from build123d import *

# Parameters (mm, degrees)
SKETCH2_W               = 3.8
SKETCH2_H               = 2.5
CUT_EXTRUDE1_DEPTH      = 10
CUT_EXTRUDE1_DEPTH_BACK = 7.25
SKETCH3_R               = 0.4
CUT_EXTRUDE2_DEPTH      = 7.25
CUT_EXTRUDE2_DEPTH_BACK = 7.25


with BuildPart() as part:
    # Sketch1 → Revolve1 (revolve)
    with BuildSketch(Plane.XY):
        with BuildLine():
            Line((0, 8.3), (0, 5.6))
            ThreePointArc((0, 5.6), (-2.071834936, 5.23939732), (-3.9, 4.2))
            Line((-3.9, 4.2), (-3.9, 0))
            Line((-3.9, 0), (-6.25, 0))
            Line((-6.25, 0), (-6.25, 4.6))
            Line((-6.25, 4.6), (-5.25, 4.6))
            ThreePointArc((-5.25, 4.6), (-3.211405456, 7.282061795), (0, 8.3))
        make_face()
    revolve(axis=Axis((0, 0, 0), (0, 1, 0)))

    # Sketch2 → Cut-Extrude1 (cut, two sides)
    with BuildSketch(Plane(origin=(0, 0, 0), x_dir=(0, 0, -1), z_dir=(1, 0, 0))) as cut_extrude1_sk:
        with Locations((0, 1.25)):
            Rectangle(SKETCH2_W, SKETCH2_H)
    extrude(amount=CUT_EXTRUDE1_DEPTH, mode=Mode.SUBTRACT)
    extrude(cut_extrude1_sk.sketch, amount=-CUT_EXTRUDE1_DEPTH_BACK, mode=Mode.SUBTRACT)

    # Sketch3 → Cut-Extrude2 (cut, two sides)
    with BuildSketch(Plane.XY) as cut_extrude2_sk:
        with Locations((0, 1.5)):
            Circle(SKETCH3_R)
    extrude(amount=CUT_EXTRUDE2_DEPTH, mode=Mode.SUBTRACT)
    extrude(cut_extrude2_sk.sketch, amount=-CUT_EXTRUDE2_DEPTH_BACK, mode=Mode.SUBTRACT)


solid = part.part
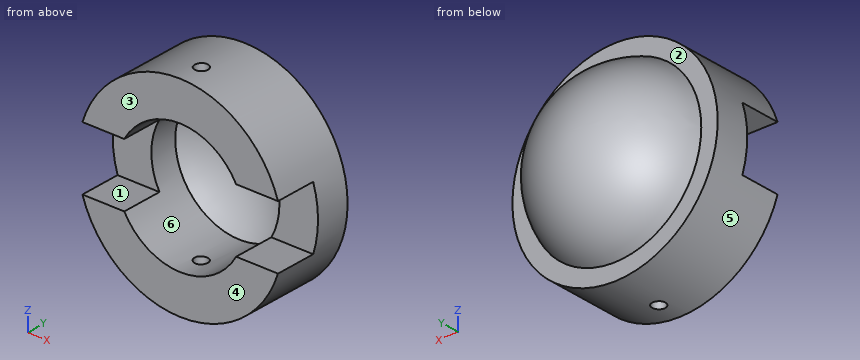
Input: part model. Units: mm. Frame: model coordinates. Face numbers are marked on the shaded views. A direction names the side the tool comes from. Coordinates: 2 decimals unless noted, no trailing zeros. Write each loop counter-clockwise with the first axis right and the second up, starting at its lowest first coordinate (ties: lowest second). Pieces come first, ordered by that corner, then holes. Notation, with made-up numbers: M 14,57 L 67,57 A18 cw 67,67 Z; hole C -28.75,29.25 d1. An arc over 180 degrees is marked long. Answer as a JSON object with one key per item and string values. Group by question number.
(1) Contact query for flat-ended pins moving along their axis: P1, Ø3, axis at x = 4.5, y = 1, coming from the +Z side; P2, Ø3, axis at x = 2.5, z = 1, coming from the +Y side; P3, Ø4, axis at y = 1, z = 0, coming from the -X side; P4, Ø3, axis at x = -5, y = 1.5, coming from the -Z side. Output: stop coordinate, or through.
(2) Set-up query: the marked faces 1, 2 and 3. Return all of +Z, -Z, +X, -X, +Y, -Y with unobstructed straight access to the full face (end or side cutting, diameter ignored); none if empty.
(3) Section D-D on z = -4.5. Output: boundary loops of the cut face in (x, y), plus the area to 3 significant figures.
(4) Section C-C on z = 0. Output: boundary loops of the cut face in (x, y).
(5) Mould query, pull axis Z, two halves, no side actions, for the marked faces 4, 5 and 6. Classes: pulls with the +Z half, pulls with the -Z half, needs draft (parallel to the pull), parting line crosses it, or undercut.
(6) Section B-B on y = 1.5. Output: boundary loops of the cut face in (x, z).
(7) Section A-A on x = 0. Output: boundary loops of the cut face in (y, z).
(8) Ray query, line 1 along Z through (x, y) = (0, 2.35); line 2 along X through (y, z) = (1.5, -4.55). Return the intervals inside material, ascending. Write a range as [from, to].
Result set:
{
 "1": {"P1": "stops at z = 5.48", "P2": "stops at y = 8.17", "P3": "stops at x = -6.25", "P4": "stops at z = -5.18"},
 "2": {"face 1": "+X, -X, -Y", "face 2": "+Y", "face 3": "+Z, -Z, +X, -X, -Y"},
 "3": {"outline": "M -4.34,0 L 4.34,0 L 4.34,4.6 L 2.7,4.6 A3.29 ccw -2.7,4.6 L -4.34,4.6 Z; hole C 0,1.5 d0.8", "area": "44.8 mm2"},
 "4": {"outline": "M -6.25,2.5 L -3.9,2.5 L -3.9,4.2 A6.13 cw 3.9,4.2 L 3.9,2.5 L 6.25,2.5 L 6.25,4.6 L 5.25,4.6 A5.57 ccw -5.25,4.6 L -6.25,4.6 Z"},
 "5": {"face 4": "needs draft", "face 5": "parting line crosses it", "face 6": "undercut"},
 "6": {"outline": "M -5.95,-1.9 A6.25 ccw -0.4,-6.24 L -0.4,-3.88 A3.9 cw -3.41,-1.9 Z; M -5.95,1.9 L -3.41,1.9 A3.9 cw -0.4,3.88 L -0.4,6.24 A6.25 ccw Z; M 0.4,-6.24 A6.25 ccw 5.95,-1.9 L 3.41,-1.9 A3.9 cw 0.4,-3.88 Z; M 0.4,3.88 A3.9 cw 3.41,1.9 L 5.95,1.9 A6.25 ccw 0.4,6.24 Z"},
 "7": {"outline": "M 0,-6.25 L 1.1,-6.25 L 1.1,-3.9 L 0,-3.9 Z; M 0,3.9 L 1.1,3.9 L 1.1,6.25 L 0,6.25 Z; M 1.9,-6.25 L 4.6,-6.25 L 4.6,-5.25 A5.57 ccw 4.6,5.25 L 4.6,6.25 L 1.9,6.25 L 1.9,3.9 L 4.2,3.9 A6.13 cw 4.2,-3.9 L 1.9,-3.9 Z"},
 "8": {"line 1": "z = [-6.25, -3.9], [3.9, 6.25]", "line 2": "x = [-4.28, -0.4], [0.4, 4.28]"}
}
